Source: CAD feature listing. Evaluate the final solid. Frame: model axes, mm. Face numbers are marked on the shaded views. A direction names the side the tool comes from. Give positions to 0.01 mm unless a question says otherwise; leave off trailing zeros. Order: outer loops, then holes, each group sorted by start corner. A loop starts at its lowest first (then second) coordinate and runs counter-clockwise, first axis right, second up.
1) Access query for the marked faces 1 and 2. Directions: +Z, -Z, +X, -X, +Y, -Y. A direction counts if a zero-diameter tool reaches every point of the face in a straight line with its end or side. Return the directions, or none.
2) Section A-A, the plane z = 59. Return loops of the section in (x, y) (1 decimal), plus the area to 3 significant figures.
3) Section C-C, the plane x = 31.5. Return loops of the section in (y, z) (3 decimals).
4) Material intervals for line 1 (X direction, y = 271.5, z = 95); line 2 (Y direction, x = -2.5, z = 63.5); line 3 (X direction, y = 91.5, z = 54.5), sorted ascending.
5) First-contact query: P1, Ø4, axis at y = 277.477, z = 41.275, coming from the +X side (1 decimal); P2, Ø9, axis at y = 144.13, z = 109.54, coming from the -X side; P3, Ø8, axis at y = 103, z = 64.5, coming from the +X side; P4, Ø6, axis at y = 60.5, z = 26.5, coming from the -X side. Flat tips, straight axial feed; report the tip coordinate or a pass-through.
6) Section B-B, the plane y = 235.5. Return loops of the section in (x, z) (3 decimals), plus the area to 3 significant figures.
Autodesk Inventor part; units mm, degrees
ref_plane "YZ Plane" through (0, 0, 0) normal (1, 0, 0) x (0, 1, 0)
ref_plane "XZ Plane" through (0, 0, 0) normal (0, 1, 0) x (-1, 0, 0)
ref_plane "XY Plane" through (0, 0, 0) normal (0, 0, 1) x (1, 0, 0)
sketch "Sketch1" plane through (0, 0, 0) normal (0, 0, 1) x (1, 0, 0)
  arc A0 (-53.3863, -0.6924) -> (55.4959, 129.0683) centre (-76.2666, 129.0683) ccw
  line L0 (-53.3863, -0.6924) -> (-231.8416, -32.1589)
  line L1 (-231.8416, -35.3829) -> (-231.8416, -32.1589)
  line L2 (-231.8416, -35.3829) -> (-52.835, -3.8192)
  arc A1 (-52.835, -3.8192) -> (58.6709, 129.0683) centre (-76.2666, 129.0683) ccw
  line L3 (58.6709, 129.0683) -> (58.6709, 290.177)
  line L4 (55.4959, 290.177) -> (58.6709, 290.177)
  line L5 (55.4959, 290.177) -> (55.4959, 129.0683)
  point P0 (0, 0)
extrude "Extrusion1" add sketch "Sketch1" along normal blind 117.475
hole "Hole1" at (55.4959, 277.477, 109.5375) direction (1, 0, 0) diameter 6.731 depth 25.4 tip angle 118
pattern_linear "Rectangular Pattern1" count 2 spacing 68.2625 along (0, 0, -1) of "Hole1"
pattern_linear "Rectangular Pattern2" count 2 spacing 133.35 along (0, -1, 0) of "Hole1"
hole "Hole2" at (-219.3346, -29.9536, 109.5375) direction (0.1736482, -0.9848078, 0) diameter 6.731 depth 25.4 tip angle 118
pattern_linear "Rectangular Pattern3" count 2 spacing 133.35 along (0.9848078, 0.1736482, 0) of "Hole2"
properties part number "GE-12071-03"
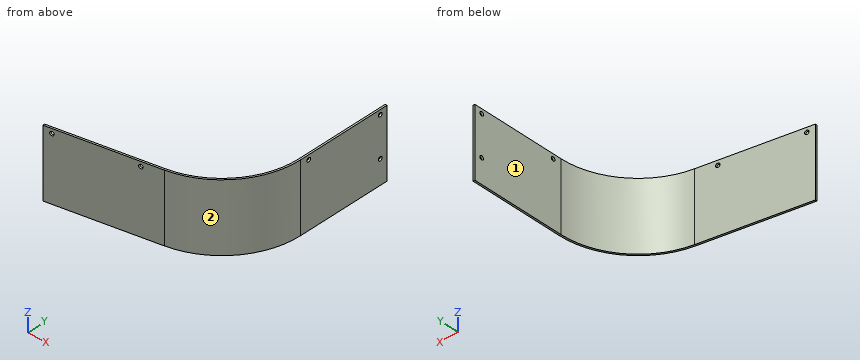
From the geometry:
1. face 1: +Z, -Z, -X, +Y
1. face 2: +Z, -Z, +X, -Y
2. outline: (-231.8, -35.4) - (-52.8, -3.8) arc R134.9 ccw to (58.7, 129.1) - (58.7, 290.2) - (55.5, 290.2) - (55.5, 129.1) arc R131.8 cw to (-53.4, -0.7) - (-231.8, -32.2) - close
2. area: 1,680 mm2
3. outline: (47.862, 0) - (53.255, 0) - (53.255, 117.475) - (47.862, 117.475) - close
4. line 1: x = 55.5 to 58.67
4. line 2: y = 16.08 to 19.89
4. line 3: x = 50.03 to 53.34
5. P1: passes through
5. P2: stops at x = 55.5
5. P3: stops at x = 56.85
5. P4: stops at x = 34.36
6. outline: (55.496, 0) - (58.671, 0) - (58.671, 117.475) - (55.496, 117.475) - close
6. area: 373 mm2
